Autodesk Inventor part; units mm, degrees
ref_plane "YZ Plane" through (0, 0, 0) normal (1, 0, 0) x (0, 1, 0)
ref_plane "XZ Plane" through (0, 0, 0) normal (0, 1, 0) x (-1, 0, 0)
ref_plane "XY Plane" through (0, 0, 0) normal (0, 0, 1) x (1, 0, 0)
sketch "Sketch5" plane through (0, 0, 0) normal (1, 0, 0) x (0, 1, 0)
  line L0 (-25.4, 38.1) -> (25.4, 38.1)
  line L1 (38.1, 25.4) -> (38.1, -25.4)
  line L2 (25.4, -38.1) -> (-25.4, -38.1)
  line L3 (-38.1, -25.4) -> (-38.1, 25.4)
  line L4 (-38.1, 38.1) -> (38.1, -38.1) construction
  line L5 (38.1, 38.1) -> (-38.1, -38.1) construction
  arc A0 (38.1, 25.4) -> (25.4, 38.1) centre (25.4, 25.4) ccw
  arc A1 (25.4, -38.1) -> (38.1, -25.4) centre (25.4, -25.4) ccw
  arc A2 (-38.1, -25.4) -> (-25.4, -38.1) centre (-25.4, -25.4) ccw
  arc A3 (-25.4, 38.1) -> (-38.1, 25.4) centre (-25.4, 25.4) ccw
  line L6 (31.75, -25.4) -> (31.75, 25.4)
  arc A4 (31.75, 25.4) -> (25.4, 31.75) centre (25.4, 25.4) ccw
  line L7 (25.4, 31.75) -> (-25.4, 31.75)
  arc A5 (-25.4, 31.75) -> (-31.75, 25.4) centre (-25.4, 25.4) ccw
  line L8 (-31.75, 25.4) -> (-31.75, -25.4)
  arc A6 (-31.75, -25.4) -> (-25.4, -31.75) centre (-25.4, -25.4) ccw
  line L9 (-25.4, -31.75) -> (25.4, -31.75)
  arc A7 (25.4, -31.75) -> (31.75, -25.4) centre (25.4, -25.4) ccw
  point P0 (0, 0)
  dimension "d6" = 76.2
  dimension "d7" = 76.2
  dimension "d8" = 12.7
  dimension "d9" = 6.35
extrude "Extrusion4" add sketch "Sketch5" along normal mid plane 304.8
sketch "Sketch7" plane through (-152.4, 0, 0) normal (-1, 0, 0) x (0, 0, 1)
  arc A0 (-38.1, -25.4) -> (-25.4, -38.1) centre (-25.4, -25.4) ccw
  line L0 (-25.4, -38.1) -> (25.4, -38.1)
  arc A1 (25.4, -38.1) -> (38.1, -25.4) centre (25.4, -25.4) ccw
  line L1 (38.1, -25.4) -> (38.1, 25.4)
  arc A2 (38.1, 25.4) -> (25.4, 38.1) centre (25.4, 25.4) ccw
  line L2 (25.4, 38.1) -> (-25.4, 38.1)
  arc A3 (-25.4, 38.1) -> (-38.1, 25.4) centre (-25.4, 25.4) ccw
  line L3 (-38.1, 25.4) -> (-38.1, -25.4)
  arc A4 (-44.45, -25.4) -> (-25.4, -44.45) centre (-25.4, -25.4) ccw
  line L4 (-25.4, -44.45) -> (25.4, -44.45)
  arc A5 (25.4, -44.45) -> (44.45, -25.4) centre (25.4, -25.4) ccw
  line L5 (44.45, -25.4) -> (44.45, 25.4)
  arc A6 (44.45, 25.4) -> (25.4, 44.45) centre (25.4, 25.4) ccw
  line L6 (25.4, 44.45) -> (-25.4, 44.45)
  arc A7 (-25.4, 44.45) -> (-44.45, 25.4) centre (-25.4, 25.4) ccw
  line L7 (-44.45, 25.4) -> (-44.45, -25.4)
  point P0 (0, 0)
extrude "Extrusion5" add sketch "Sketch7" against normal blind 15.875
fillet "Fillet1" radius 6.35 16 edges at (-152.4, 38.8704, -38.8704) (-152.4, 0, -44.45) (-152.4, -38.8704, -38.8704) (-152.4, -44.45, 0) (-152.4, -38.8704, 38.8704) (-152.4, 0, 44.45) (-152.4, 38.8704, 38.8704) (-152.4, 44.45, 0) (-136.525, 38.8704, 38.8704) (-136.525, 0, 44.45) (-136.525, -38.8704, 38.8704) (-136.525, -44.45, 0) (-136.525, -38.8704, -38.8704) (-136.525, 0, -44.45) (-136.525, 38.8704, -38.8704) (-136.525, 44.45, 0)
sketch "Sketch8" plane through (0, 0, 0) normal (0, 0, 1) x (1, 0, 0)
  circle A0 centre (-88.9, 0) radius 8.255
  line L0 (-152.4, 25.4) -> (-152.4, -25.4)
  point P0 (0, 0)
  dimension "d15" = 63.5
  dimension "d16" = 16.51
extrude "Extrusion6" cut sketch "Sketch8" along normal through all both and the other way through all
pattern_linear "Rectangular Pattern1" count 2 spacing 76.2 along (1, 0, 0) of "Extrusion6"
properties part number "Front Hitch Model-1_Base Tube-2" material "SS304"
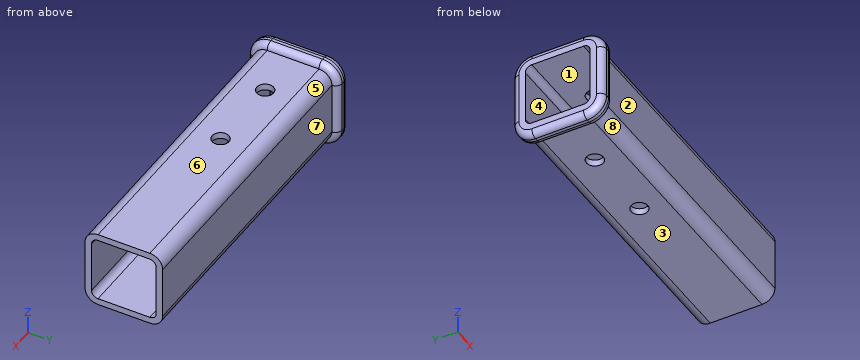
Part model, mm, in its own coordinate system. Face numbers are marked on the shaded views. A direction names the side the tool comes from. Coordinates: 2 decimals unless noted, no trailing zeros. Loops run counter-clockwise (first coordinate to the right, second up) from the corner with the lowest first, then second, coordinate; pieces in that order, holes last. Notation, with made-up numbers: M 59,64 L 68,64 A19 cw 68,78 Z; hole C -6,35 d4. An arc over 180 degrees is marked long. Use a Markdown table: item, result. Add a question column.
Q1. Probe L1, parallel to X at y = 0, z = 36 (3 decimals); L2, parallel to Y at x = -17.5, z = -19. List the from-to ranges inside material, lowest first.
Q2. Which spindle directions (+Z, -Z, +X, -X, +Y, -Y) get a long thin tool onto all of the face, cutting with end or side? Do the marked faces 4, 5, 6, 7 and 8. Say none if no direction does.
Q3. Mould opens along Z. For the marked faces 1, 2 and 3 say: +Z half, -Z half, draft (parallel to the pull), parting line (faces both ways), or undercut.
Q4. Pin check, flat tips, straight feed: P1, Ø15, axis at x = -49, y = 7.5, coming from the -Z side; P2, Ø5, axis at x = 43, z = -29, coming from the -Y side; P3, Ø4, axis at x = -67, y = -35.5, coming from the -Z side. Stop position of each tip, or through.
Q5. Cut at B-B (x = -12.7). Write the cut outline in (y, z) (3 decimals), and give its area (3 significant figures).
Q6. Cut at C-C (y = 0). Give the number of separate pieces and of enclosed holes in the cut face, and give its area (3 significant figures).
Worked out:
| question | item | result |
|---|---|---|
| 1 | L1 | x = -152.4 to -97.155, -80.645 to -20.955, -4.445 to 152.4 |
| 1 | L2 | y = -38.1 to -31.75, 31.75 to 38.1 |
| 2 | face 4 | +X, -X |
| 2 | face 5 | +Z, +X, +Y |
| 2 | face 6 | +Z, +X, +Y, -Y |
| 2 | face 7 | +Z, -Z, +X, +Y |
| 2 | face 8 | -Z, +X, -Y |
| 3 | face 1 | undercut |
| 3 | face 2 | draft |
| 3 | face 3 | -Z half |
| 4 | P1 | stops at z = -38.1 |
| 4 | P2 | stops at y = -38.05 |
| 4 | P3 | stops at z = -35.18 |
| 5 | outline | M -38.1,-25.4 A12.7 ccw -25.4,-38.1 L -8.255,-38.1 L -8.255,-31.75 L -25.4,-31.75 A6.35 cw -31.75,-25.4 L -31.75,25.4 A6.35 cw -25.4,31.75 L -8.255,31.75 L -8.255,38.1 L -25.4,38.1 A12.7 ccw -38.1,25.4 Z; M 8.255,-38.1 L 25.4,-38.1 A12.7 ccw 38.1,-25.4 L 38.1,25.4 A12.7 ccw 25.4,38.1 L 8.255,38.1 L 8.255,31.75 L 25.4,31.75 A6.35 cw 31.75,25.4 L 31.75,-25.4 A6.35 cw 25.4,-31.75 L 8.255,-31.75 Z |
| 5 | area | 1,460 mm2 |
| 6 | separate pieces | 6 |
| 6 | enclosed holes | 0 |
| 6 | area | 3,620 mm2 |
